```python
from build123d import *

# Parameters (mm, degrees)
EXTRUDE_1_DEPTH     = 4
SKETCH_4_R          = 0.5
CUT_EXTRUDE_1_DEPTH = 7
CUT_EXTRUDE_4_DEPTH = 3
CUT_EXTRUDE_5_DEPTH = 3
CUT_EXTRUDE_6_DEPTH = 3


with BuildPart() as part:
    # 草图3 → 凸台-拉伸1 (new body)
    with BuildSketch(Plane.XY):
        with BuildLine():
            Line((0, -2), (20, -2))
            Line((20, -2), (20, 2))
            Line((20, 2), (0, 2))
            ThreePointArc((0, 2), (-2, 0), (0, -2))
        make_face()
    extrude(amount=EXTRUDE_1_DEPTH)

    # 草图4 → 切除-拉伸1 (cut)
    with BuildSketch(Plane(origin=(20, 0, 0), x_dir=(0, 0, -1), z_dir=(1, 0, 0))):
        with Locations((-2, 0)):
            Circle(SKETCH_4_R)
    extrude(amount=-CUT_EXTRUDE_1_DEPTH, mode=Mode.SUBTRACT)

    # 草图5 → 切除-拉伸4 (cut)
    with BuildSketch(Plane.XY.offset(4)):
        with BuildLine():
            Line((-0.866025404, 0.5), (-1.366025404, 0.5))
            Line((-1.366025404, 0.5), (-1.366025404, 1.460812992))
            ThreePointArc((-1.366025404, 1.460812992), (-2, 0), (-1.366025404, -1.460812992))
            Line((-1.366025404, -1.460812992), (-1.366025404, -0.5))
            Line((-1.366025404, -0.5), (-0.866025404, -0.5))
            ThreePointArc((-0.866025404, -0.5), (1, 0), (-0.866025404, 0.5))
        make_face()
    extrude(amount=-CUT_EXTRUDE_4_DEPTH, mode=Mode.SUBTRACT)

    # 草图6 → 切除-拉伸5 (cut)
    with BuildSketch(Plane.XY.offset(1)):
        with BuildLine():
            Line((-1.366025404, 0.5), (-1.366025404, -0.5))
            Line((-1.366025404, -0.5), (-1.366025404, -1.460812992))
            ThreePointArc((-1.366025404, -1.460812992), (-2, 0), (-1.366025404, 1.460812992))
            Line((-1.366025404, 1.460812992), (-1.366025404, 0.5))
        make_face()
    extrude(amount=-CUT_EXTRUDE_5_DEPTH, mode=Mode.SUBTRACT)

    # 草图7 → 切除-拉伸6 (cut)
    with BuildSketch(Plane.XY.offset(4)):
        with BuildLine():
            Line((10.527261775, -0.595306745), (10.328163394, -1.053956758))
            ThreePointArc((10.328163394, -1.053956758), (9.423448211, -1.281600523), (8.828273079, -2))
            Line((8.828273079, -2), (9.917489301, -2))
            Line((9.917489301, -2), (11.007645162, -2))
            Line((11.007645162, -2), (11.619083211, -2))
            ThreePointArc((11.619083211, -2), (11.462926396, -1.705172003), (11.24546342, -1.45215352))
            Line((11.24546342, -1.45215352), (11.444561801, -0.993503507))
            ThreePointArc((11.444561801, -0.993503507), (11.728957062, 0.917300026), (10.527261775, -0.595306745))
        make_face()
    extrude(amount=-CUT_EXTRUDE_6_DEPTH, mode=Mode.SUBTRACT)


solid = part.part
```
Geometry check sheet. Reference: the model listing, model coordinates, mm. A direction names the side the tool comes from. Coordinates: 2 decimals unless noted, no trailing zeros. Order: outer loops, then holes, each group sorted by start corner. A loop starts at its lowest first (then second) coordinate and runs counter-clockwise, first axis right, second up. Notation, with made-up numbers: M 62,68 L 66,68 A32 cw 66,100 Z; hole C 74.25,-39 d9. An arc over 180 degrees is marked long. One line per question, with ' | ' between items. Start each with the question number.
Item 1: Gauge pin test, flat ends, axial feed: pin 1 (0.5 mm diameter, centred on x = -1, z = 3, fed in from +Y); pin 2 (1.6 mm diameter, centred on x = 0, y = 0, fed in from +Z); pin 3 (0.8 mm diameter, centred on y = 0, z = 2, fed in from +X). Record the tip position at first contact, or that the pin passes through.
Item 2: Set-up check for faces 4 (the flat face through (-1.366, -1, 2)), 5 (the flat face through (0, 0, 1)), 6 (the cylindrical face through (9.435, -1.275, 2.521)): record each of +Z, -Z, +X, -X, +Y, -Y from which the full face is reachable in a straight line by a thin tool's end or side.
Item 3: Cross-section at C-C on y = 0. Enter the section's corners in (x, z).
Item 4: Material ranges on L1, parallel to X at y = 0.55, z = 1.8; L2, parallel to Y at x = 18.5, z = 2; L3, parallel to X at y = 0, z = 3.1, recorded low to high. Write a range as [from, to].
Item 5: Cross-section at B-B on x = 17.75. Enter the section's corners in (y, z).
Item 6: Cross-section at A-A on z = 2. Enter the section's corners in (x, y), then the cut area to 3 significant figures.
Item 7: Cross-section at D-D on z = 3.25. Enter the section's corners in (x, y), then the cut area to 3 significant figures.
Item 8: Draft check along X on faces 1 (the flat face through (13, 0, 2)), 2 (the cylindrical face through (1, 0, 3)), 3 (the cylindrical face through (16.5, -0.3, 2.4)). Enter one of: pulls with the +X half, pulls with the -X half, needs draft (parallel to the pull), parting line crosses it, or undercut.
Findings:
1) pin 1: stops at y = 1.85 | pin 2: stops at z = 1 | pin 3: stops at x = 13
2) face 4: +Z, -Z, -X, +Y, -Y | face 5: +Z | face 6: +Z, -Y
3) outline: M -1.37,0 L 20,0 L 20,1.5 L 13,1.5 L 13,2.5 L 20,2.5 L 20,4 L 12.33,4 L 12.33,1 L 10.33,1 L 10.33,4 L 1,4 L 1,1 L -1.37,1 Z
4) L1: x = [-1.37, -0.84], [0.84, 10.5], [12.17, 20] | L2: y = [-2, -0.5], [0.5, 2] | L3: x = [1, 10.33], [12.33, 20]
5) outline: M -2,0 L 2,0 L 2,4 L -2,4 Z; hole C 0,2 d1
6) outline: M -1.37,-1.46 A2 ccw 0,-2 L 8.83,-2 A1.5 cw 10.33,-1.05 L 10.53,-0.6 A1 cw long 11.44,-0.99 L 11.25,-1.45 A1.5 cw 11.62,-2 L 20,-2 L 20,-0.5 L 13,-0.5 L 13,0.5 L 20,0.5 L 20,2 L 0,2 A2 ccw -1.37,1.46 L -1.37,0.5 L -0.87,0.5 A1 cw long -0.87,-0.5 L -1.37,-0.5 Z | area: 69.0 mm²
7) outline: M -1.37,-1.46 A2 ccw 0,-2 L 8.83,-2 A1.5 cw 10.33,-1.05 L 10.53,-0.6 A1 cw long 11.44,-0.99 L 11.25,-1.45 A1.5 cw 11.62,-2 L 20,-2 L 20,2 L 0,2 A2 ccw -1.37,1.46 L -1.37,0.5 L -0.87,0.5 A1 cw long -0.87,-0.5 L -1.37,-0.5 Z | area: 76.0 mm²
8) face 1: pulls with the +X half | face 2: undercut | face 3: needs draft
